from build123d import *

# Parameters (mm, degrees)
BOSS_EXTRUDE1_DEPTH      = 100
SKETCH2_R                = 7.5
CUT_EXTRUDE2_DEPTH       = 100
SKETCH3_R                = 7.5
CUT_EXTRUDE3_DEPTH       = 100
CUT_EXTRUDE4_DEPTH       = 100
SKETCH5_R                = 7.5
CUT_EXTRUDE5_DEPTH       = 20
BOSS_EXTRUDE2_DEPTH      = 5
BOSS_EXTRUDE2_DEPTH_BACK = 105
SKETCH7_R                = 6
CUT_EXTRUDE6_START       = -35
CUT_EXTRUDE6_DEPTH       = 35
FILLET1_R                = 1


with BuildPart() as part:
    # Sketch1 → Boss-Extrude1 (new body)
    with BuildSketch(Plane.XY):
        Polygon((0, 0), (85, 0), (85, 10), (47.715081247, 10), (47.715081247, 25), (62.715081247, 25), (62.715081247, 45), (32.715081247, 45), (0, 25), align=None)
    extrude(amount=-BOSS_EXTRUDE1_DEPTH)

    # Sketch2 → Cut-Extrude2 (cut)
    with BuildSketch(Plane(origin=(0, 10, 0), x_dir=(1, 0, 0), z_dir=(0, 1, 0))):
        with Locations(Location((65, 15, 0), (0, 0, 180))):
            Circle(SKETCH2_R)
        with BuildLine():
            Line((47.5, 65), (47.5, 35))
            ThreePointArc((47.5, 35), (55, 27.5), (62.5, 35))
            Line((62.5, 35), (62.5, 65))
            ThreePointArc((62.5, 65), (55, 72.5), (47.5, 65))
        make_face()
    extrude(amount=-CUT_EXTRUDE2_DEPTH, mode=Mode.SUBTRACT)

    # Sketch3 → Cut-Extrude3 (cut)
    with BuildSketch(Plane(origin=(0, 10, 0), x_dir=(1, 0, 0), z_dir=(0, 1, 0))):
        with Locations(Location((55, 85, 0), (0, 0, 193.754716541))):
            Circle(SKETCH3_R)
    extrude(amount=-CUT_EXTRUDE3_DEPTH, mode=Mode.SUBTRACT)

    # Sketch4 → Cut-Extrude4 (cut)
    with BuildSketch(Plane(origin=(0, 10, 0), x_dir=(1, 0, 0), z_dir=(0, 1, 0))):
        Polygon((75, 0), (85, 10), (85, 0), align=None)
    extrude(amount=-CUT_EXTRUDE4_DEPTH, mode=Mode.SUBTRACT)

    # Sketch5 → Cut-Extrude5 (cut)
    with BuildSketch(Plane(origin=(-11.125485694, 18.19855842, 0), x_dir=(0.8531953684822633, 0.5215914715564423, 0), z_dir=(-0.5215914715564423, 0.8531953684822633, 0))):
        with Locations((32.211879404, 0)):
            Circle(SKETCH5_R)
    extrude(amount=-CUT_EXTRUDE5_DEPTH, mode=Mode.SUBTRACT)

    # Sketch7 → Boss-Extrude2 (add, two sides: drawn at the far end of the back side and taken through both)
    with BuildSketch(Plane.XY.offset(-BOSS_EXTRUDE2_DEPTH_BACK)):
        with Locations((62.715081247, 35)):
            Circle(SKETCH7_R)
    extrude(amount=BOSS_EXTRUDE2_DEPTH + BOSS_EXTRUDE2_DEPTH_BACK)

    # Sketch8 → Cut-Extrude6 (cut)
    with BuildSketch(Plane(origin=(0, 45, 0), x_dir=(1, 0, 0), z_dir=(0, 1, 0)).offset(CUT_EXTRUDE6_START)):
        Polygon((62.715081247, 90), (42.715081247, 90), (42.715081247, 22.5), (72.715081247, 22.5), (72.715081247, 90), align=None)
    extrude(amount=CUT_EXTRUDE6_DEPTH, mode=Mode.SUBTRACT)

    # Fillet1
    fillet1_edges = [part.edges().sort_by_distance(p)[0] for p in [
        (55, 10, -27.5),
        (55, 10, -72.5),
        (62.5, 10, -50),
        (47.5, 10, -50),
        (72.5, 10, -15),
        (62.284918753, 10, -86.783243887),
    ]]
    fillet(fillet1_edges, radius=FILLET1_R)


solid = part.part
The model under review builds one solid part; all positions refer to its coordinate system, in mm. A direction names the side the tool comes from. Round coordinates to 2 decimals unless told otherwise and drop trailing zeros. Order: outer loops, then holes, each group sorted by start corner. A loop starts at its lowest first (then second) coordinate and runs counter-clockwise, first axis right, second up. Notation, with made-up numbers: (46, 1) - (62, 1) arc R25 cw to (62, 36) - close; hole circle Ø8 at (48.25, -33.5). An arc over 180 degrees is marked (long way). Use one line per item in the form item = value.
Q1. Clearance check with flat-ended pins moving along their axes: P1, Ø10, axis at x = 23.5, y = 5, coming from the -Z side; P2, Ø3, axis at y = 25.5, z = -41.5, coming from the +X side; P3, Ø1.2, axis at y = 27.5, z = -5.5, coming from the +X side. State where each tip first meets the part, or that it passes through.
Response values:
P1 = -100
P2 = 42.72
P3 = 62.72
Q2. Add section C-C on y = 7.5. Give the boundary of the cut face in (x, z), then the cut area to 3 significant figures.
Response values:
outline = (0, -100) - (85, -100) - (85, -10) - (75, 0) - (0, 0) - close; hole circle Ø15 at (55, -85); hole (47.5, -65) arc R7.5 ccw to (62.5, -65) - (62.5, -35) arc R7.5 ccw to (47.5, -35) - close; hole circle Ø15 at (65, -15)
area = 7,470 mm^2
Q3. Add section B-B on x = 55. Give the boundary of the cut face in (y, z), then the cut area to 3 significant figures.
Response values:
outline = (0, -100) - (10, -100) - (10, -93.5) arc R1 ccw to (9, -92.5) - (0, -92.5) - close; (0, -77.5) - (9, -77.5) arc R1 ccw to (10, -76.5) - (10, -73.5) arc R1 ccw to (9, -72.5) - (0, -72.5) - close; (0, -27.5) - (9, -27.5) arc R1 ccw to (10, -26.5) - (10, 0) - (0, 0) - close; (25, -100) - (45, -100) - (45, -90) - (25, -90) - close; (25, -22.5) - (45, -22.5) - (45, 0) - (25, 0) - close
area = 1,050 mm^2
Q4. Mouldability with a two-part tool opening along X and no side actions: class faces 1 (the flat face through (85, 5, -54)), 2 (the flat face through (62.5, 5, -50)), 3 (the flat face through (55, 25, -11)), 4 (the cylindrical face through (70.5, 4.6, -9.9)) as pulls with the +X half, pulls with the -X half, needs draft (parallel to the pull), parting line crosses it, or undercut.
Response values:
face_1 = pulls with the +X half
face_2 = undercut
face_3 = needs draft
face_4 = undercut
Q5. Add section A-A on z = -62. Give the boundary of the cut face in (x, y).
Response values:
outline = (0, 0) - (47.5, 0) - (47.5, 9) arc R1 ccw to (46.5, 10) - (42.72, 10) - (42.72, 45) - (32.72, 45) - (0, 25) - close; (62.5, 0) - (85, 0) - (85, 10) - (63.5, 10) arc R1 ccw to (62.5, 9) - close
Q6. Tool access review of faces 5 (the flat face through (55, 25, -95)), 6 (the flat face through (42.715, 27, -57)), 7 (the cylindrical face through (54.84, 4.56, -27.5)): name each direction out of +Z, -Z, +X, -X, +Y, -Y from which nothing blocks a thin tool from reaching the whole face with its end or side.
Response values:
face_5 = +Z, -Z, +X
face_6 = +X, +Y
face_7 = +Y, -Y
Q7. To check wall thickness, follow line 1 (Z direction, x = 54.5, y = 3.5); line 2 (X direction, y = 6.75, z = -85); line 3 (Z direction, x = 65, y = 6). State the ranges of each line that lie inside material, in increasing order.
Response values:
line_1 = -100 to -92.48, -77.52 to -72.48, -27.52 to 0
line_2 = 0 to 47.5, 62.5 to 85
line_3 = -100 to -22.5, -7.5 to 0
Q8. Add section D-D on x = 38. Give the boundary of the cut face in (y, z), then the cut area to 3 significant figures.
Response values:
outline = (0, -100) - (45, -100) - (45, 0) - (0, 0) - close
area = 4,500 mm^2
